from build123d import *

# Parameters (mm, degrees)
SKETCH1_W           = 250
SKETCH1_H           = 16
BOSS_EXTRUDE1_DEPTH = 14
SKETCH2_R           = 7
CUT_EXTRUDE1_DEPTH  = 148.715171273
CUT_EXTRUDE3_DEPTH  = 148.715171273
SKETCH4_R           = 7
BOSS_EXTRUDE2_DEPTH = 14
SKETCH5_R           = 7
BOSS_EXTRUDE3_DEPTH = 40


with BuildPart() as part:
    # Sketch1 → Boss-Extrude1 (new body)
    with BuildSketch(Plane.XY):
        with Locations((17.628205128, 27.790598291)):
            Rectangle(SKETCH1_W, SKETCH1_H)
    extrude(amount=BOSS_EXTRUDE1_DEPTH)

    # Sketch2 → Cut-Extrude1 (cut, through all)
    with BuildSketch(Plane.XY.offset(14)):
        with Locations((126.832264356, 27.518873536)):
            Circle(SKETCH2_R)
    extrude(amount=-CUT_EXTRUDE1_DEPTH, mode=Mode.SUBTRACT)

    # Sketch3 → Cut-Extrude3 (cut, through all)
    with BuildSketch(Plane.XY.offset(14)):
        with BuildLine():
            Line((142.628205128, 19.790598291), (134.612843431, 19.790598291))
            ThreePointArc((134.612843431, 19.790598291), (137.92655193, 27.790598291), (134.612843431, 35.790598291))
            Line((134.612843431, 35.790598291), (142.628205128, 35.790598291))
            Line((142.628205128, 35.790598291), (142.628205128, 19.790598291))
        make_face()
    extrude(amount=-CUT_EXTRUDE3_DEPTH, mode=Mode.SUBTRACT)

    # Sketch4 → Boss-Extrude2 (add)
    with BuildSketch(Plane.XY.offset(14)):
        with Locations(Location((-96.531660716, 27.264616337, 0), (0, 0, 180))):
            Circle(SKETCH4_R)
    extrude(amount=BOSS_EXTRUDE2_DEPTH)

    # Sketch5 → Boss-Extrude3 (add)
    with BuildSketch(Plane.XY.offset(28)):
        with Locations(Location((-96.531660716, 27.264616337, 0), (0, 0, 180))):
            Circle(SKETCH5_R)
    extrude(amount=BOSS_EXTRUDE3_DEPTH)


solid = part.part
Source: CAD feature listing. Evaluate the final solid. Frame: model axes, mm. A direction names the side the tool comes from. Round coordinates to 2 decimals unless told otherwise and drop trailing zeros. Write each loop counter-clockwise with the first axis right and the second up, starting at its lowest first coordinate (ties: lowest second). Pieces come first, ordered by that corner, then holes. Notation, with made-up numbers: M 55,-20 L 70,-20 A15 ccw 70,-1 Z; hole C 54,30.5 d5. An arc over 180 degrees is marked long. One line per item, written item: value. Start each with the question number.
Item 1: Section query A-A (y = 24). Return the cut outline in (x, z), plus the area to 3 significant figures.
Item 2: Mould query, pull axis Y, two halves, no side actions, for faces 3 (the flat face through (12, 35.791, 7)), 4 (the cylindrical face through (133.3, 24.84, 7.1)), 5 (the cylindrical face through (137.926, 27.666, 7.098)), 6 (the flat face through (14, 28, 14)). Classes: pulls with the +Y half, pulls with the -Y half, needs draft (parallel to the pull), parting line crosses it, or undercut.
Item 3: Pin query (flat end, axial travel): pin 1 (8.5 mm diameter, centred on x = 126.83, y = 27.52, fed in from +Z); pin 2 (5 mm diameter, centred on x = 53.5, y = 26, fed in from +Z); pin 3 (1 mm diameter, centred on y = 26, z = 32, fed in from +X); pin 4 (5 mm diameter, centred on x = 110.5, y = 29, fed in from -Z). Return the tip coordinate at first contact, or that it passes through.
Item 4: Section query C-C (z = 61). Return the cut outline in (x, y).
Item 5: Section query B-B (x = 50). Return the cut outline in (y, z).
Item 6: Ray query, L1, parallel to Z at x = -13, y = 26.5; L2, parallel to X at y = 22.25, z = 9.5; L3, parallel to X at y = 24.5, z = 5. Return the intervals inside material, ascending. Write a range as from..to.
Item 7: Set-up query: faces 1 (the flat face through (12, 19.791, 7)), 2 (the cylindrical face through (-102.998, 29.946, 40.622)). Return all of +Z, -Z, +X, -X, +Y, -Y with unobstructed straight access to the full face (end or side cutting, diameter ignored); none if empty.
Result set:
1. outline: M -107.37,0 L 120.78,0 L 120.78,14 L -90.34,14 L -90.34,68 L -102.72,68 L -102.72,14 L -107.37,14 Z; M 132.88,0 L 137.27,0 L 137.27,14 L 132.88,14 Z
1. area: 3,920 mm²
2. face 3: pulls with the +Y half
2. face 4: undercut
2. face 5: parting line crosses it
2. face 6: needs draft
3. pin 1: passes through
3. pin 2: stops at z = 14
3. pin 3: stops at x = -89.57
3. pin 4: stops at z = 0
4. outline: C -96.53,27.26 d14
5. outline: M 19.79,0 L 35.79,0 L 35.79,14 L 19.79,14 Z
6. L1: z = 0..14
6. L2: x = -107.37..122.22, 131.44..136.48
6. L3: x = -107.37..120.52, 133.15..137.44
7. face 1: +Z, -Z, +X, -X, -Y
7. face 2: +Z
